```python
from build123d import *

# Parameters (mm, degrees)
CYLINDER005_R        = 1.5
CYLINDER005_DEPTH    = 10
BOX022_W             = 10
BOX022_H             = 7.5
BOX022_DEPTH         = 15
FILLET002008005014_R = 3.4


with BuildPart() as cylinder005:
    # Cylinder005 → Cylinder005 (new body)
    with BuildSketch(Plane(origin=(90, 10, 28.25), x_dir=(0, 0, -1), z_dir=(1, 0, 0))):
        Circle(CYLINDER005_R)
    extrude(amount=CYLINDER005_DEPTH)


with BuildPart() as fillet002008005014:
    # Box022 → Box022 (new body)
    with BuildSketch(Plane(origin=(90, 6.25, 17), x_dir=(1, 0, 0), z_dir=(0, 0, 1))):
        with Locations((5, 3.75)):
            Rectangle(BOX022_W, BOX022_H)
    extrude(amount=BOX022_DEPTH)

    # Cut001005: cut Cylinder005
    add(cylinder005.part, mode=Mode.SUBTRACT)

    # Fillet002008005014
    fillet002008005014_edges = [fillet002008005014.edges().sort_by_distance(p)[0] for p in [
        (95, 6.25, 32),
        (95, 13.75, 32),
    ]]
    fillet(fillet002008005014_edges, radius=FILLET002008005014_R)


with BuildPart() as fillet002008005014_1:
    # Fillet002008005014 placement: moved
    add(fillet002008005014.part.moved(Location((0, 0, 3.5))))


solid = fillet002008005014_1.part
```
Geometry check sheet. Reference: the model listing, model coordinates, mm. Coordinates: 2 decimals unless noted, no trailing zeros. Loops run counter-clockwise (first coordinate to the right, second up) from the corner with the lowest first, then second, coordinate; pieces in that order, holes last. Notation, with made-up numbers: (59, 81) -> (73, 81) arc R9 cw to (73, 95) -> close; hole circle Ø2 at (-17.5, 37.5). An arc over 180 degrees is marked (long way). Put each result on its own line as item: value.
1) Gauge pin test, flat end, axial feed: pin 1 Ø2.5 at (y, z) = (10, 31.75) entering from +X. Record the tip position at first contact, or that the pin passes through.
Result set:
pin 1: passes through
2) Cross-section at A-A on z = 31.75. Record the boundary of the cut face in (x, y).
Result set:
outline: (90, 6.25) -> (100, 6.25) -> (100, 8.5) -> (90, 8.5) -> close; (90, 11.5) -> (100, 11.5) -> (100, 13.75) -> (90, 13.75) -> close
3) Thickness scan on line 1 (Y direction, x = 97.25, z = 31.75); line 2 (Y direction, x = 93, z = 31.25); line 3 (Z direction, x = 92, y = 13). Record the ranges inside material, lowest first.
Result set:
line 1: y = 6.25 to 8.5, 11.5 to 13.75
line 2: y = 6.25 to 8.59, 11.41 to 13.75
line 3: z = 20.5 to 34.23
4) Cross-section at C-C on x = 90.75. Record the boundary of the cut face in (y, z).
Result set:
outline: (6.25, 20.5) -> (13.75, 20.5) -> (13.75, 32.1) arc R3.4 ccw to (10.35, 35.5) -> (9.65, 35.5) arc R3.4 ccw to (6.25, 32.1) -> close; hole circle Ø3 at (10, 31.75)
5) Cross-section at B-B on y = 10. Record the boundary of the cut face in (x, z).
Result set:
outline: (90, 20.5) -> (100, 20.5) -> (100, 30.25) -> (90, 30.25) -> close; (90, 33.25) -> (100, 33.25) -> (100, 35.5) -> (90, 35.5) -> close
6) Cross-section at D-D on y = 7.25. Record the boundary of the cut face in (x, z), plus the area to 3 significant figures.
Result set:
outline: (90, 20.5) -> (100, 20.5) -> (100, 34.51) -> (90, 34.51) -> close
area: 140 mm^2
7) Release check for a two-part mould opening along Y. For faces 1 (the flat face through (95, 6.25, 26)), 2 (the cylindrical face through (94.93, 9.09, 32.94)), 3 (the flat face through (95, 13.75, 26)) record: released by +Y, released by -Y, zero draft, split by the parting line, or undercut.
Result set:
face 1: released by -Y
face 2: undercut
face 3: released by +Y
